Input: part model. Units: mm. Frame: model coordinates. A direction names the side the tool comes from. Give positions to 0.01 mm unless a question says otherwise; leave off trailing zeros. Loops run counter-clockwise (first coordinate to the right, second up) from the corner with the lowest first, then second, coordinate; pieces in that order, holes last. Notation, with made-up numbers: (-12, -15) - (13, -15) arc R27 cw to (13, 14) - close; hole circle Ø6 at (34, 36). An arc over 180 degrees is marked (long way). One line per item, written item: value.
from build123d import *

# Parameters (mm, degrees)
EXTRUDE_1_DEPTH     = 76
CUT_EXTRUDE_1_DEPTH = 52
SHELL_2_T           = -1.75
SKETCH_7_R          = 2.5
CUT_EXTRUDE_3_DEPTH = 49.861876587
SKETCH_7_2_R        = 2.5
CUT_EXTRUDE_4_DEPTH = 3


with BuildPart() as part:
    # Sketch 1 → Extrude 1 (new body)
    with BuildSketch(Plane.XY):
        Polygon((11.494238236, 7.609934935), (-16.411750997, 7.609934935), (-39.505761764, -32.390065065), (11.494238236, -32.390065065), align=None)
    extrude(amount=EXTRUDE_1_DEPTH)

    # Sketch 2 → Cut-Extrude 1 (cut, through all)
    with BuildSketch(Plane(origin=(11.494238236, 0, 0), x_dir=(0, 0, -1), z_dir=(1, 0, 0))):
        Polygon((-57, 7.609934935), (-76, -32.390065065), (-76, 7.609934935), align=None)
        Polygon((-19, 7.609934935), (0, -32.390065065), (0, 7.609934935), align=None)
    extrude(amount=-CUT_EXTRUDE_1_DEPTH, mode=Mode.SUBTRACT)

    # Shell 2
    shell_2_openings = [part.faces().sort_by_distance(p)[0] for p in [
        (-14.005761764, -32.390065065, 38),
    ]]
    offset(amount=SHELL_2_T, openings=shell_2_openings, kind=Kind.INTERSECTION)

    # Sketch 7 → Cut-Extrude 3 (cut, through all)
    with BuildSketch(Plane(origin=(1.902483734, 7.100165955, 0), x_dir=(0.965925826, -0.258819045, 0), z_dir=(0.258819045, 0.965925826, 0))):
        with Locations((-1.969596093, -38)):
            Circle(SKETCH_7_R)
    extrude(amount=-CUT_EXTRUDE_3_DEPTH, mode=Mode.SUBTRACT)

    # Sketch 7_2 → Cut-Extrude 4 (cut)
    with BuildSketch(Plane(origin=(1.902483734, 7.100165955, 0), x_dir=(0.965925826, -0.258819045, 0), z_dir=(0.258819045, 0.965925826, 0))):
        with Locations((-1.969596093, -38)):
            Circle(SKETCH_7_2_R)
    extrude(amount=CUT_EXTRUDE_4_DEPTH, mode=Mode.SUBTRACT)


solid = part.part
Item 1: Draft query along X for faces 1 (the face through (11.494, -17, 37)), 2 (the face through (-5, 7.61, 38)), 3 (the face through (-28.742, -17.247, 37.495)), 4 (the face through (-8.292, -12.997, 64.851)). Return one class per face: pulls with the +X half, pulls with the -X half, needs draft (parallel to the pull), parting line crosses it, or undercut.
Verdict:
face 1: pulls with the +X half
face 2: needs draft
face 3: undercut
face 4: undercut
Item 2: Section B-B, the plane z = 53. Output: boundary loops of the cut face in (x, y).
Verdict:
outline: (-39.51, -32.39) - (-37.49, -32.39) - (-15.4, 5.86) - (9.74, 5.86) - (9.74, -32.39) - (11.49, -32.39) - (11.49, 7.61) - (-16.41, 7.61) - close
Item 3: Material intervals for L1, parallel to Y at x = 3, z = 47.5; L2, parallel to X at y = -10.5, z = 58; L3, parallel to X at y = -17.5, z = 37.5, sorted ascending.
Verdict:
L1: y = 5.86 to 7.61
L2: x = -26.87 to -24.85, 9.74 to 11.49
L3: x = -30.91 to -28.89, 9.74 to 11.49
Item 4: Section A-A, the plane y = 3. Output: boundary loops of the cut face in (x, z).
Verdict:
outline: (-19.07, 16.81) - (11.49, 16.81) - (11.49, 59.19) - (-19.07, 59.19) - close; hole (-17.05, 18.75) - (9.74, 18.75) - (9.74, 57.25) - (-17.05, 57.25) - close
Item 5: Section C-C, the plane x = -7.5. Output: boundary loops of the cut face in (y, z), and give its area (3 significant figures).
Verdict:
outline: (-32.39, 0) - (7.61, 19) - (7.61, 57) - (-32.39, 76) - (-32.39, 74.06) - (5.86, 55.89) - (5.86, 20.11) - (-32.39, 1.94) - close
area: 216 mm^2
Item 6: Access query for faces 5 (the face through (-5, 5.86, 38)), 6 (the face through (-7.982, -12.11, 66.367)). Directions: +Z, -Z, +X, -X, +Y, -Y. A direction counts if a zero-diameter tool reaches every point of the face in a straight line with its end or side. Return the directions, or none.
Verdict:
face 5: -Y
face 6: +Z, +X, -X, +Y
Item 7: Pin query (flat end, axial travel): P1, Ø1.5, axis at x = -10, y = -21, coming from the -Z side; P2, Ø2, axis at x = -13, y = -20.5, coming from the +Z side; P3, Ø2, axis at x = -3, y = -16, coming from the +Z side; P4, Ø20, axis at x = 3.5, z = 43, coming from the -Y side. Return the tip coordinate at first contact, or that it passes through.
Verdict:
P1: stops at z = 5.05
P2: stops at z = 70.83
P3: stops at z = 68.69
P4: stops at y = -32.39
Item 8: Section D-D, the plane y = -3. Output: boundary loops of the cut face in (x, z).
Verdict:
outline: (-22.54, 13.96) - (11.49, 13.96) - (11.49, 62.04) - (-22.54, 62.04) - close; hole (-20.52, 15.9) - (9.74, 15.9) - (9.74, 60.1) - (-20.52, 60.1) - close
